from build123d import *

# Parameters (mm, degrees)
EXTRUDE_1_DEPTH = 50
FILLET_1_R      = 0.4


with BuildPart() as part:
    # Эскиз1 → Бобышка-Вытянуть1 (new body)
    with BuildSketch(Plane.XY):
        with BuildLine():
            Line((17.5, -4.25), (17.5, -0.5))
            Line((17.5, -0.5), (16.616025404, -0.5))
            ThreePointArc((16.616025404, -0.5), (14.75, 0), (16.616025404, 0.5))
            Line((16.616025404, 0.5), (17.5, 0.5))
            Line((17.5, 0.5), (17.5, 4.25))
            ThreePointArc((17.5, 4.25), (16.75, 5), (16, 4.25))
            Line((16, 4.25), (16, 2.25))
            Line((16, 2.25), (13.5, 2.25))
            Line((13.5, 2.25), (13.5, 4.5))
            ThreePointArc((13.5, 4.5), (13, 5), (12.5, 4.5))
            Line((12.5, 4.5), (12.5, 1))
            Line((12.5, 1), (10, 1))
            Line((10, 1), (10, 4.5))
            ThreePointArc((10, 4.5), (9.5, 5), (9, 4.5))
            Line((9, 4.5), (9, 1))
            Line((9, 1), (-9, 1))
            Line((-9, 1), (-9, 4.5))
            ThreePointArc((-9, 4.5), (-9.5, 5), (-10, 4.5))
            Line((-10, 4.5), (-10, 1))
            Line((-10, 1), (-12.5, 1))
            Line((-12.5, 1), (-12.5, 4.5))
            ThreePointArc((-12.5, 4.5), (-13, 5), (-13.5, 4.5))
            Line((-13.5, 4.5), (-13.5, 2.25))
            Line((-13.5, 2.25), (-16, 2.25))
            Line((-16, 2.25), (-16, 4.25))
            ThreePointArc((-16, 4.25), (-16.75, 5), (-17.5, 4.25))
            Line((-17.5, 4.25), (-17.5, 0.5))
            Line((-17.5, 0.5), (-16.616025404, 0.5))
            ThreePointArc((-16.616025404, 0.5), (-14.75, 0), (-16.616025404, -0.5))
            Line((-16.616025404, -0.5), (-17.5, -0.5))
            Line((-17.5, -0.5), (-17.5, -4.25))
            ThreePointArc((-17.5, -4.25), (-16.75, -5), (-16, -4.25))
            Line((-16, -4.25), (-16, -2.25))
            Line((-16, -2.25), (-13.5, -2.25))
            Line((-13.5, -2.25), (-13.5, -4.5))
            ThreePointArc((-13.5, -4.5), (-13, -5), (-12.5, -4.5))
            Line((-12.5, -4.5), (-12.5, -1))
            Line((-12.5, -1), (-10, -1))
            Line((-10, -1), (-10, -4.5))
            ThreePointArc((-10, -4.5), (-9.5, -5), (-9, -4.5))
            Line((-9, -4.5), (-9, -1))
            Line((-9, -1), (-6.5, -1))
            Line((-6.5, -1), (-6.5, -4.5))
            ThreePointArc((-6.5, -4.5), (-6, -5), (-5.5, -4.5))
            Line((-5.5, -4.5), (-5.5, -1))
            Line((-5.5, -1), (5.5, -1))
            Line((5.5, -1), (5.5, -4.5))
            ThreePointArc((5.5, -4.5), (6, -5), (6.5, -4.5))
            Line((6.5, -4.5), (6.5, -1))
            Line((6.5, -1), (9, -1))
            Line((9, -1), (9, -4.5))
            ThreePointArc((9, -4.5), (9.5, -5), (10, -4.5))
            Line((10, -4.5), (10, -1))
            Line((10, -1), (12.5, -1))
            Line((12.5, -1), (12.5, -4.5))
            ThreePointArc((12.5, -4.5), (13, -5), (13.5, -4.5))
            Line((13.5, -4.5), (13.5, -2.25))
            Line((13.5, -2.25), (16, -2.25))
            Line((16, -2.25), (16, -4.25))
            ThreePointArc((16, -4.25), (16.75, -5), (17.5, -4.25))
        make_face()
    extrude(amount=EXTRUDE_1_DEPTH)

    # Скругление1
    fillet_1_edges = [part.edges().sort_by_distance(p)[0] for p in [
        (-17.5, -0.5, 25),
        (-16.616025404, -0.5, 25),
        (-16.616025404, 0.5, 25),
        (-17.5, 0.5, 25),
        (17.5, 0.5, 25),
        (16.616025404, 0.5, 25),
        (16.616025404, -0.5, 25),
        (17.5, -0.5, 25),
    ]]
    fillet(fillet_1_edges, radius=FILLET_1_R)


solid = part.part
The model under review builds one solid part; all positions refer to its coordinate system, in mm. A direction names the side the tool comes from. Give positions to 0.01 mm unless a question says otherwise; leave off trailing zeros. Order: outer loops, then holes, each group sorted by start corner. A loop starts at its lowest first (then second) coordinate and runs counter-clockwise, first axis right, second up. Notation, with made-up numbers: M 64,15.25 L 112,15.25 A24 cw 112,51.25 Z; hole C -5.75,42 d2. An arc over 180 degrees is marked long. Answer in a Markdown table with one row per item. Add a question column.
1. Add section B-B on x = 6. State the section outline as (y, z) points, plus the area to 3 significant figures.
2. Add section C-C on y = 0. State the section outline as (x, z) points.
3. To check wall thickness, follow line 1 along X through (y, z) = (-1.5, 15); line 2 along X through (y, z) = (2, 8); line 3 along X through (y, z) = (3.75, 15). State the ranges of each line that lie inside material, in increasing order.
4. For pin 1 Ø4 at (x, y) = (9, 3) entering from -Z; pin 2 Ø3 at (x, z) = (15, 18) entering from -Y, all flat-tipped, find the tip position at first contact; note any pin that passes through.
5. Add section A-A on y = -3. Count the separate pieces of the cut face and the enclosed holes in it, plus the area to 3 significant figures.
6. Mouldability with a two-part tool opening along Y and no side actions: class faces 1 (the cylindrical face through (-14.75, 0.03, 24.65)), 2 (the cylindrical face through (-9.5, 5, 24.6)), 3 (the cylindrical face through (16.7, -5, 24.6)) as released by +Y, released by -Y, zero draft, split by the parting line, or undercut.
7. Machinability: for faces 4 (the flat face through (-9, -3, 25)), 5 (the flat face through (0, 0, 0)), 6 (the flat face through (10, 3, 25)), which of the approach directions +Z, -Z, +X, -X, +Y, -Y give a long, thin tool a straight path to every point of the face, cutting with its end or side? Answer none if there is none.
The answers:
| question | item | result |
|---|---|---|
| 1 | outline | M -5,0 L 1,0 L 1,50 L -5,50 Z |
| 1 | area | 300 mm2 |
| 2 | outline | M -14.75,0 L 14.75,0 L 14.75,50 L -14.75,50 Z |
| 3 | line 1 | -17.5 to -12.5, -10 to -9, -6.5 to -5.5, 5.5 to 6.5, 9 to 10, 12.5 to 17.5 |
| 3 | line 2 | -17.5 to -12.5, -10 to -9, 9 to 10, 12.5 to 17.5 |
| 3 | line 3 | -17.5 to -16, -13.5 to -12.5, -10 to -9, 9 to 10, 12.5 to 13.5, 16 to 17.5 |
| 4 | pin 1 | z = 0 |
| 4 | pin 2 | y = -4.96 |
| 5 | separate pieces | 8 |
| 5 | enclosed holes | 0 |
| 5 | area | 450 mm2 |
| 6 | face 1 | undercut |
| 6 | face 2 | released by +Y |
| 6 | face 3 | released by -Y |
| 7 | face 4 | +Z, -Z, -Y |
| 7 | face 5 | -Z, +X, -X, +Y, -Y |
| 7 | face 6 | +Z, -Z, +Y |
